For this review, take the finished solid that the model builds, in its own axes (mm). Face numbers are marked on the shaded views. A direction names the side the tool comes from. Round coordinates to 2 decimals unless told otherwise and drop trailing zeros. Order: outer loops, then holes, each group sorted by start corner. A loop starts at its lowest first (then second) coordinate and runs counter-clockwise, first axis right, second up. Notation, with made-up numbers: M -27.5,83 L -23.5,83 A25 cw -23.5,103 Z; hole C 83,19.5 d2. An arc over 180 degrees is marked long. Use a Markdown table: item, result.
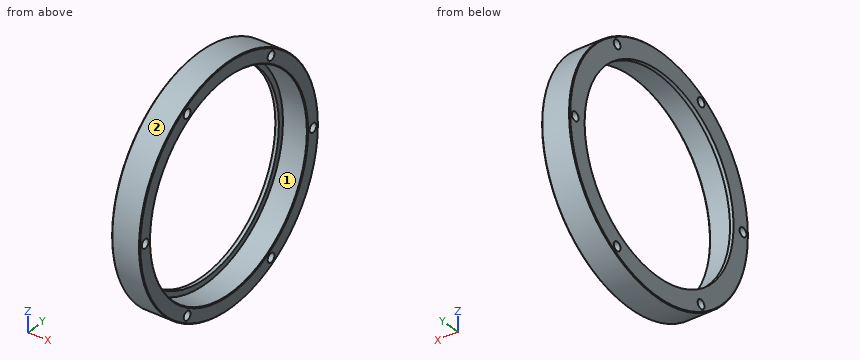
from build123d import *

# Parameters (mm, degrees)
HOLE_WIZARD_M3_1_D       = 2.5
PATTERN_CIRCULAR_1_COUNT = 6
CHAMFER_1_SIZE           = 0.2


with BuildPart() as part:
    # 草图1 → 旋转1 (revolve)
    with BuildSketch(Plane.XY):
        Polygon((0, 27.5), (0, 33), (8, 33), (8, 29), (1, 29), (1, 27.5), align=None)
    revolve(axis=Axis((0, 0, 0), (1, 0, 0)))

    # M3 螺纹孔1 (through all)
    with Locations(Plane(origin=(8, 0, 0), x_dir=(0, 0, -1), z_dir=(1, 0, 0))):
        with Locations((0, 31)):
            hole_wizard_m3_1 = Hole(HOLE_WIZARD_M3_1_D / 2)

    # 阵列(圆周)1: M3 螺纹孔1 ×6 about axis
    pattern_circular_1_axis = Axis((0, 0, 0), (1, 0, 0))
    for i in range(1, PATTERN_CIRCULAR_1_COUNT):
        add(hole_wizard_m3_1.rotate(pattern_circular_1_axis, i * 360 / PATTERN_CIRCULAR_1_COUNT), mode=Mode.SUBTRACT)

    # 倒角1
    chamfer_1_edges = [part.edges().sort_by_distance(p)[0] for p in [
        (8, -29, 0),
        (8, -33, 0),
        (0, -33, 0),
    ]]
    chamfer(chamfer_1_edges, length=CHAMFER_1_SIZE)


solid = part.part
Q1. Add section C-C (y = -15.5). Give the number of separate pieces and of enclosed holes in the cut face, then the cut area to 3 significant figures.
Determined:
| item | result |
|---|---|
| separate pieces | 4 |
| enclosed holes | 0 |
| area | 37.4 mm^2 |
Q2. Clearance check with flat-ended pins moving along their axes: pin 1 (3 mm diameter, centred on y = 31, z = 0, fed in from -X); pin 2 (2 mm diameter, centred on x = 6, y = 13.5, fed in from +Z); pin 3 (4 mm diameter, centred on x = 4, y = 16, fed in from -Z); pin 4 (1 mm diameter, centred on x = 3, z = 16, fed in from -Y). State where each tip first meets the part, or that it passes through.
Determined:
| item | result |
|---|---|
| pin 1 | stops at x = 0 |
| pin 2 | stops at z = 30.54 |
| pin 3 | stops at z = -29.88 |
| pin 4 | stops at y = -29.13 |
Q3. Add section A-A (y = 0). Write out the cut boundary in (x, z).
Determined:
| item | result |
|---|---|
| outline | M 0,-32.8 L 0.2,-33 L 7.8,-33 L 8,-32.8 L 8,-29.2 L 7.8,-29 L 1,-29 L 1,-27.5 L 0,-27.5 Z; M 0,27.5 L 1,27.5 L 1,29 L 7.8,29 L 8,29.2 L 8,32.8 L 7.8,33 L 0.2,33 L 0,32.8 Z |
Q4. Add section B-B (x = 4.25). Write out the cut boundary in (y, z).
Determined:
| item | result |
|---|---|
| outline | C 0,0 d66; hole C -31,0 d2.5; hole C 0,0 d58; hole C -15.5,-26.85 d2.5; hole C -15.5,26.85 d2.5; hole C 15.5,-26.85 d2.5; hole C 15.5,26.85 d2.5; hole C 31,0 d2.5 |
Q5. Machinability: for the marked faces 1 and 2, which of the approach directions +Z, -Z, +X, -X, +Y, -Y give a long, thin tool a straight path to every point of the face, cutting with its end or side? Answer none if there is none.
Determined:
| item | result |
|---|---|
| face 1 | +X |
| face 2 | +X, -X |
Q6. Wall thickness on line 1 along Z through (x, y) = (6, 0); line 2 along Z through (x, y) = (7.5, -25); line 3 along Y through (x, z) = (7.5, 22): over which ranges is each line inside the solid? List them lowest first. Write a range as [from, to].
Determined:
| item | result |
|---|---|
| line 1 | z = [-33, -29], [29, 33] |
| line 2 | z = [-21.54, -14.7], [14.7, 21.54] |
| line 3 | y = [-24.6, -18.89], [18.89, 24.6] |
